For this review, use the dimensioned drawing (mm, ordinates from the lowest corner) and the shaded views. A direction names the side the tool comes from. Round coordinates to 2 decimals unless told otherwise and drop trailing zeros. Loops run counter-clockwise (first coordinate to the right, second up) from the corner with the lowest first, then second, coordinate; pieces in that order, holes last. Notation, with made-up numbers: M -28.75,49.25 L 23.25,49.25 A10 cw 23.25,54.25 Z; hole C -21,3 d5. An arc over 180 degrees is marked long. One line per item, written item: value. Start each with the question number.
Item 1: For line 1 along Y through (x, z) = (2.5, 7.5); line 2 along Z through (x, y) = (15.25, 5.5); line 3 along X through (y, z) = (22, 6.75), list the stretches that pass through material, from the lowest coordinate up.
Item 2: For the marked faces 1 and 2, list the 3-axis set-ups (+Z, -Z, +X, -X, +Y, -Y) from which the entire face can be reached by the end or side of a thin tool; tool diameter is ignored.
Item 3: We need section D-D (x = 5.25). Write out the cut boundary in (y, z).
Item 4: We need section B-B (x = 18). Write out the cut boundary in (y, z).
Item 5: We need section C-C (y = 22.5). Write out the cut boundary in (x, z).
Item 6: Clearance check with flat-ended pins moving along their axes: pin 1 (8 mm diameter, centred on x = 5.5, y = 14, fed in from -Z); pin 2 (3 mm diameter, centred on x = 14.5, y = 25.5, fed in from +Z); pin 3 (3 mm diameter, centred on y = 37.5, z = 2.5, fed in from -X); pin 4 (2 mm diameter, centred on y = 38.5, z = 5, fed in from -X). State where each tip first meets the part, or that it passes through.
Item 7: We need section A-A (z = 7). Write out the cut boundary in (x, y).
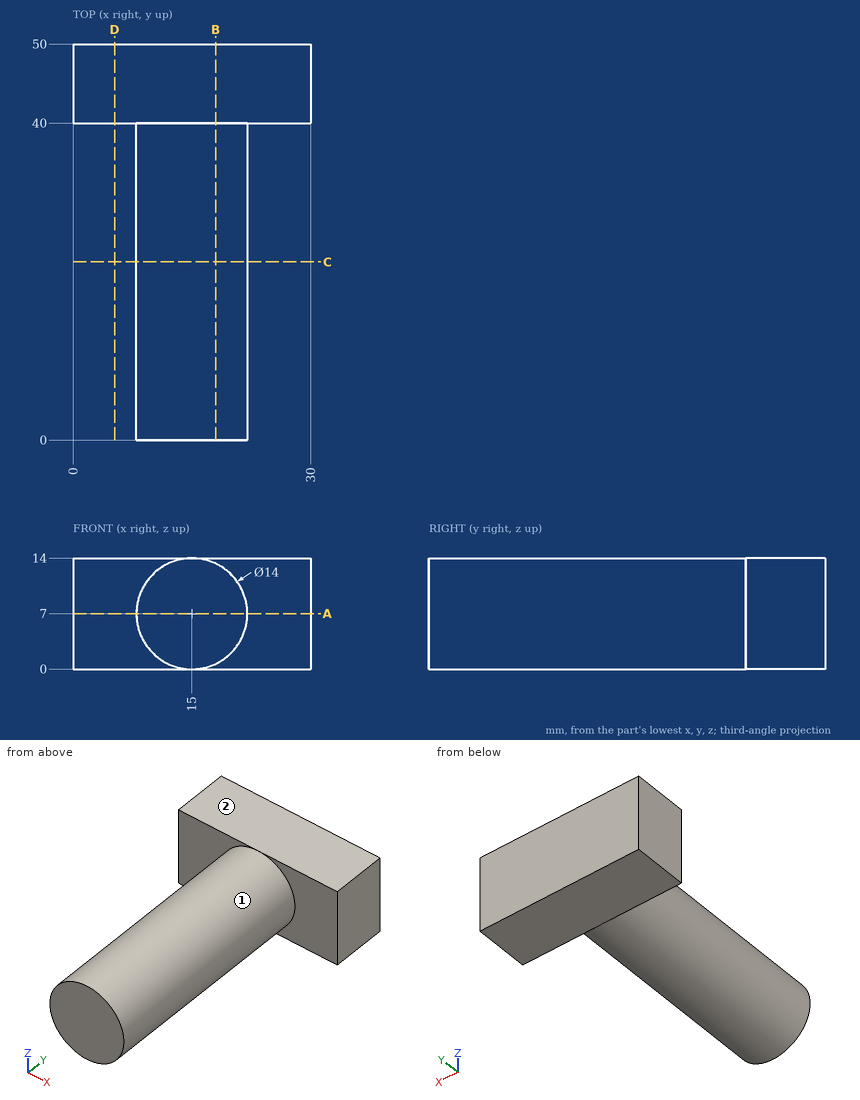
A:
1. line 1: 40 to 50
1. line 2: 0 to 14
1. line 3: 8 to 22
2. face 1: -Y
2. face 2: +Z, +X, -X, +Y, -Y
3. outline: M 40,0 L 50,0 L 50,14 L 40,14 Z
4. outline: M 0,0.68 L 40,0.68 L 40,0 L 50,0 L 50,14 L 40,14 L 40,13.32 L 0,13.32 Z
5. outline: C 15,7 d14
6. pin 1: z = 2.67
6. pin 2: z = 14
6. pin 3: x = 8.68
6. pin 4: x = 8.07
7. outline: M 0,40 L 8,40 L 8,0 L 22,0 L 22,40 L 30,40 L 30,50 L 0,50 Z
